```python
from build123d import *

# Parameters (mm, degrees)
SKETCH1_R           = 12.7
BOSS_EXTRUDE1_DEPTH = 12.7


with BuildPart() as part:
    # Sketch1 → Boss-Extrude1 (new body)
    with BuildSketch(Plane(origin=(0, 0, 0), x_dir=(1, 0, 0), z_dir=(0, 1, 0))):
        with BuildLine():
            Line((-177.80483956, -180.970122773), (-177.80483956, -34.920560393))
            Line((-177.80483956, -34.920560393), (177.79516044, -34.920560393))
            Line((177.79516044, -34.920560393), (177.79516044, -503.170122773))
            Line((177.79516044, -503.170122773), (499.99516044, -180.970122773))
            Line((499.99516044, -180.970122773), (499.99516044, 496.829877227))
            Line((499.99516044, 496.829877227), (177.795656663, 174.63037345))
            Line((177.795656663, 174.63037345), (177.795656663, 34.887353965))
            Line((177.795656663, 34.887353965), (10.941991643, 34.887353965))
            Line((10.941991643, 34.887353965), (10.941991643, 327.760499625))
            ThreePointArc((10.941991643, 327.760499625), (0.004607764, 391.44950084), (-10.950678316, 327.76357658))
            Line((-10.950678316, 327.76357658), (-10.950678316, 34.887353965))
            Line((-10.950678316, 34.887353965), (-177.804343337, 34.887353965))
            Line((-177.804343337, 34.887353965), (-177.804343337, 496.829877227))
            Line((-177.804343337, 496.829877227), (-500.00483956, 174.629381004))
            Line((-500.00483956, 174.629381004), (-500.00483956, -503.170122773))
            Line((-500.00483956, -503.170122773), (-177.80483956, -180.970122773))
        make_face()
        Polygon((-461.454447779, -145.049098288), (-203.204343337, 122.90730747), (-203.204343337, 9.487353965), (-203.20483956, -9.520560393), (-203.20483956, -145.049098288), align=None, mode=Mode.SUBTRACT)
        Polygon((-203.204343337, 164.10835652), (-474.60483956, 164.10835652), (-203.204343337, 435.508852743), align=None, mode=Mode.SUBTRACT)
        Polygon((-474.60483956, 138.70835652), (-214.240958944, 138.70835652), (-474.60483956, -130.828873379), align=None, mode=Mode.SUBTRACT)
        Polygon((-474.60483956, -170.449098288), (-203.20483956, -170.449098288), (-474.60483956, -441.849098288), align=None, mode=Mode.SUBTRACT)
        Polygon((474.59516044, 9.487353965), (474.594664217, -9.520560393), (474.594664217, -145.049098288), (223.497797401, -145.049098288), (474.59516044, 115.721361844), align=None, mode=Mode.SUBTRACT)
        Polygon((474.594664217, -170.449098288), (203.194664217, -441.849098288), (203.194664217, -170.449098288), align=None, mode=Mode.SUBTRACT)
        Polygon((203.194664217, -122.149307614), (203.194664217, 138.70835652), (453.645393175, 138.70835652), align=None, mode=Mode.SUBTRACT)
        Polygon((203.194664217, 164.10835652), (474.59516044, 435.508852743), (474.59516044, 164.10835652), align=None, mode=Mode.SUBTRACT)
        Circle(SKETCH1_R, mode=Mode.SUBTRACT)
    extrude(amount=BOSS_EXTRUDE1_DEPTH)


solid = part.part
```
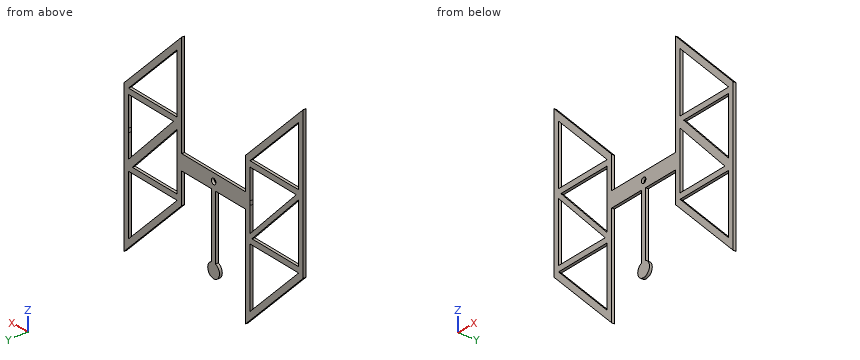
CAD build for the part. Positions are in the model's coordinates, mm. Coordinates: 2 decimals unless noted, no trailing zeros. Order: outer loops, then holes, each group sorted by start corner. A loop starts at its lowest first (then second) coordinate and runs counter-clockwise, first axis right, second up.
(1) Drill centre lines: L1, parallel to Z at x = 0, y = 3.75; L2, parallel to X at y = 5.75, z = 0; L3, parallel to Z at x = 281, y = 11. Where is each one in solid material? Low to high.
Solution:
L1: z = -391.45 to -12.7, 12.7 to 34.92
L2: x = -500 to -474.6, -348.23 to -321.66, -203.2 to -12.7, 12.7 to 203.19, 320.47 to 363.17, 474.59 to 500
L3: z = -277.83 to -241.91, -164.11 to -138.71, 41.11 to 85.33, 145.05 to 170.45, 364.04 to 399.97
(2) Pin check, flat tips, straight feed: pin 1 Ø1 at (x, y) = (-106, 5) entering from -Z; pin 2 Ø4 at (y, z) = (9, -258.5) entering from -X; pin 3 Ø6.5 at (x, y) = (369.5, 7) entering from +Z. Stop position of each tip, or through.
Solution:
pin 1: stops at z = -34.89
pin 2: stops at x = -418.13
pin 3: stops at z = 314.72
(3) Saw through at B-B, the plane z = 397. Write the cut outline in (x, y).
Solution:
outline: (-500, 0) - (-474.6, 0) - (-474.6, 12.7) - (-500, 12.7) - close; (-429.76, 0) - (-393.83, 0) - (-393.83, 12.7) - (-429.76, 12.7) - close; (177.8, 0) - (203.19, 0) - (203.19, 12.7) - (177.8, 12.7) - close; (248.04, 0) - (283.97, 0) - (283.97, 12.7) - (248.04, 12.7) - close
(4) Saw through at D-D, the plane z = 66. Write the cut outline in (x, y).
Solution:
outline: (-500, 0) - (-474.6, 0) - (-474.6, 12.7) - (-500, 12.7) - close; (-411.98, 0) - (-385.27, 0) - (-385.27, 12.7) - (-411.98, 12.7) - close; (-203.2, 0) - (-177.8, 0) - (-177.8, 12.7) - (-203.2, 12.7) - close; (177.8, 0) - (203.19, 0) - (203.19, 12.7) - (177.8, 12.7) - close; (257.1, 0) - (299.61, 0) - (299.61, 12.7) - (257.1, 12.7) - close; (474.59, 0) - (500, 0) - (500, 12.7) - (474.59, 12.7) - close
(5) Saw through at A-A, the plane x = -235.5. Write the cut outline in (y, z), and give its area (3 significant figures).
Solution:
outline: (0, -439.13) - (12.7, -439.13) - (12.7, -403.21) - (0, -403.21) - close; (0, -164.11) - (12.7, -164.11) - (12.7, -138.71) - (0, -138.71) - close; (0, -116.7) - (12.7, -116.7) - (12.7, -89.4) - (0, -89.4) - close; (0, 145.05) - (12.7, 145.05) - (12.7, 170.45) - (0, 170.45) - close; (0, 202.74) - (12.7, 202.74) - (12.7, 238.67) - (0, 238.67) - close
area: 1,900 mm2
(6) Saw through at C-C, the plane z = -100. Write the cut outline in (x, y).
Solution:
outline: (-500, 0) - (-474.6, 0) - (-474.6, 12.7) - (-500, 12.7) - close; (-251.63, 0) - (-225.28, 0) - (-225.28, 12.7) - (-251.63, 12.7) - close; (-203.2, 0) - (-177.8, 0) - (-177.8, 12.7) - (-203.2, 12.7) - close; (-10.95, 0) - (10.94, 0) - (10.94, 12.7) - (-10.95, 12.7) - close; (177.8, 0) - (203.19, 0) - (203.19, 12.7) - (177.8, 12.7) - close; (416.48, 0) - (459.46, 0) - (459.46, 12.7) - (416.48, 12.7) - close; (474.6, 0) - (500, 0) - (500, 12.7) - (474.6, 12.7) - close
